Check sheet for the modelled part. Datum: model origin and axes. Units: mm. Face numbers are marked on the shaded views. A direction names the side the tool comes from. Give positions to 0.01 mm unless a question says otherwise; leave off trailing zeros. Loops run counter-clockwise (first coordinate to the right, second up) from the corner with the lowest first, then second, coordinate; pieces in that order, holes last. Notation, with made-up numbers: M 71.5,-27.75 L 126.5,-27.75 A6 ccw 126.5,-17.75 Z; hole C 23,-39.75 d7. An arc over 180 degrees is marked long. Put each result on its own line as item: value. Start each with the question number.
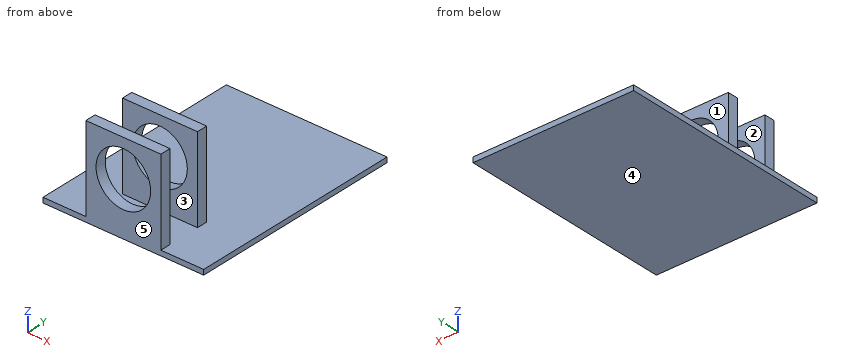
```python
from build123d import *

# Parameters (mm, degrees)
F0_W     = 35
F0_H     = 40
F0_R     = 12.75
F1_DEPTH = 100
F2_W     = 15
F2_H     = 40
F2_W_2   = 75
F3_DEPTH = 22.5


with BuildPart() as f1:
    # F0 (on Front) → F1 (new body)
    with BuildSketch(Plane.XZ):
        with Locations((0, 20)):
            Rectangle(F0_W, F0_H)
        with Locations((0, 22.6)):
            Circle(F0_R, mode=Mode.SUBTRACT)
        Polygon((-17.5, 0), (-37.5, 0), (-37.5, -2.4), (37.5, -2.4), (37.5, 0), (17.5, 0), align=None)
    extrude(amount=F1_DEPTH)

    # F2 (on Right) → F3 (cut, symmetric)
    with BuildSketch(Plane.YZ):
        with Locations((-87.5, 20)):
            Rectangle(F2_W, F2_H)
        with Locations((-37.5, 20)):
            Rectangle(F2_W_2, F2_H)
    extrude(amount=F3_DEPTH, both=True, mode=Mode.SUBTRACT)


solid = f1.part
```
Q1. Depth check by flat-ended pin: P1, Ø1.5, axis at y = -77.5, z = 23, coming from the +X side; P2, Ø2, axis at x = 9.5, z = 5, coming from the +Y side; P3, Ø22.5, axis at x = 4.5, y = -42, coming from the +Z side; P4, Ø17.5, axis at x = 2.5, z = 16.5, coming from the -Y side. Enter the tip coordinate at first touch or a pass-through.
Q2. Access from +Z, -Z, +X, -X, +Y, -Y to the whole of each face (thin tool, end or side, straight path). Record for the marked faces 1 and 2.
Q3. Mould release check, pull along Y, two halves, no side actions. Record for the marked faces 3, 4 and 5: pulls with the +Y half, pulls with the -Y half, needs draft (parallel to the pull), parting line crosses it, or undercut.
Q4. Section check B-B, the plane z = 5. Record the cut outline in (x, y), then the cut area to 3 significant figures.
Q5. Section check D-D, the plane x = -15. Record the cut outline in (y, z), then the cut area to 3 significant figures.
Q6. Thickness scan on line 1 along Y through (x, z) = (-7.5, 9); line 2 along X through (y, z) = (-96, 22); line 3 along Z through (x, y) = (0, -76). Record the ranges inside material, lowest first. Write a range as [from, to].
Q7. Section check A-A, the plane z = 22.6. Record the cut outline in (x, y), then the cut area to 3 significant figures.
Q8. Section check C-C, the plane x = 0. Record the cut outline in (y, z), then the cut area to 3 significant figures.
Found:
1. P1: stops at x = 17.5
1. P2: stops at y = -75
1. P3: stops at z = 0
1. P4: stops at y = -100
2. face 1: +Z, +X, -X, +Y
2. face 2: +Z, +X, -X
3. face 3: undercut
3. face 4: needs draft
3. face 5: pulls with the -Y half
4. outline: M -17.5,-100 L 17.5,-100 L 17.5,-95 L -17.5,-95 Z; M -17.5,-80 L 17.5,-80 L 17.5,-75 L -17.5,-75 Z
4. area: 350 mm^2
5. outline: M -100,-2.4 L 0,-2.4 L 0,0 L -75,0 L -75,40 L -80,40 L -80,0 L -95,0 L -95,40 L -100,40 Z
5. area: 640 mm^2
6. line 1: y = [-100, -95], [-80, -75]
6. line 2: x = [-17.5, -12.74], [12.74, 17.5]
6. line 3: z = [-2.4, 9.85], [35.35, 40]
7. outline: M -17.5,-100 L -12.75,-100 L -12.75,-95 L -17.5,-95 Z; M -17.5,-80 L -12.75,-80 L -12.75,-75 L -17.5,-75 Z; M 12.75,-100 L 17.5,-100 L 17.5,-95 L 12.75,-95 Z; M 12.75,-80 L 17.5,-80 L 17.5,-75 L 12.75,-75 Z
7. area: 95.0 mm^2
8. outline: M -100,-2.4 L 0,-2.4 L 0,0 L -75,0 L -75,9.85 L -80,9.85 L -80,0 L -95,0 L -95,9.85 L -100,9.85 Z; M -100,35.35 L -95,35.35 L -95,40 L -100,40 Z; M -80,35.35 L -75,35.35 L -75,40 L -80,40 Z
8. area: 385 mm^2
